The model under review builds one solid part; all positions refer to its coordinate system, in mm. A direction names the side the tool comes from. Round coordinates to 2 decimals unless told otherwise and drop trailing zeros. Order: outer loops, then holes, each group sorted by start corner. A loop starts at its lowest first (then second) coordinate and runs counter-clockwise, first axis right, second up.
```python
from build123d import *

# Parameters (mm, degrees)
SKETCH1_W                  = 44.45
SKETCH1_H                  = 60
CUT_EXTRUDE1_DEPTH         = 50
F_4_CLEARANCE_HOLE1_D      = 3.3
F_4_CLEARANCE_HOLE1_DEPTH  = 8
F_2_CLEARANCE_HOLE1_REACH  = 117.544
F_2_CLEARANCE_HOLE1_BORE_R = 1.25
F_2_CLEARANCE_HOLE2_REACH  = 117.544
F_2_CLEARANCE_HOLE2_BORE_R = 1.25


with BuildPart() as part:
    # Sketch1 → Revolve1 (revolve)
    with BuildSketch(Plane.XZ, mode=Mode.PRIVATE) as revolve1_sk:
        with Locations((22.225, 30)):
            Rectangle(SKETCH1_W, SKETCH1_H)
    revolve(revolve1_sk.sketch.rotate(Axis((0, 0, 60), (0, 0, -1)), 180), axis=Axis((0, 0, 60), (0, 0, -1)))

    # Sketch2 → Cut-Extrude1 (cut)
    with BuildSketch(Plane(origin=(0, 0, 0), x_dir=(-1, 0, 0), z_dir=(0, 0, -1))):
        with BuildLine():
            Line((43.7241638, 8), (43.7241638, -8))
            ThreePointArc((43.7241638, -8), (44.45, 0), (43.7241638, 8))
        make_face()
    extrude(amount=-CUT_EXTRUDE1_DEPTH, mode=Mode.SUBTRACT)

    # Sketch3 → Cut-Revolve1 (revolve, cut)
    with BuildSketch(Plane.XZ, mode=Mode.PRIVATE) as cut_revolve1_sk:
        Polygon((37.5, 60), (0, 60), (0, 0), (37.5, 0), (37.5, 20.5), (32, 20.5), (32, 39.5), (37.5, 39.5), align=None)
    revolve(cut_revolve1_sk.sketch.rotate(Axis((0, 0, 60), (0, 0, -1)), 180), axis=Axis((0, 0, 60), (0, 0, -1)), mode=Mode.SUBTRACT)

    # #4 Clearance Hole1
    with Locations(Plane.XY.offset(60)):
        with Locations((28.991378029, 28.991378029), (0, 41), (-28.991378029, 28.991378029), (-41, 0), (-28.991378029, -28.991378029), (0, -41), (28.991378029, -28.991378029), (41, 0)):
            Hole(F_4_CLEARANCE_HOLE1_D / 2, depth=F_4_CLEARANCE_HOLE1_DEPTH)

    # #2 Clearance Hole1 bore → #2 Clearance Hole1 (cut, up to next)
    with BuildSketch(Plane.ZY.offset(43.7241638), mode=Mode.PRIVATE) as f_2_clearance_hole1_sk1:
        with Locations((15.584748033, 5.15)):
            Circle(F_2_CLEARANCE_HOLE1_BORE_R)
    f_2_clearance_hole1_tool1 = extrude(f_2_clearance_hole1_sk1.sketch, amount=-F_2_CLEARANCE_HOLE1_REACH, mode=Mode.PRIVATE) & part.part
    add(f_2_clearance_hole1_tool1.solids().sort_by_distance((-43.724164, 5.15, 15.584748))[0], mode=Mode.SUBTRACT)

    # #2 Clearance Hole2 bore → #2 Clearance Hole2 (cut, up to next)
    with BuildSketch(Plane.ZY.offset(43.7241638), mode=Mode.PRIVATE) as f_2_clearance_hole2_sk1:
        with Locations((37.834748033, -5.05)):
            Circle(F_2_CLEARANCE_HOLE2_BORE_R)
    f_2_clearance_hole2_tool1 = extrude(f_2_clearance_hole2_sk1.sketch, amount=-F_2_CLEARANCE_HOLE2_REACH, mode=Mode.PRIVATE) & part.part
    add(f_2_clearance_hole2_tool1.solids().sort_by_distance((-43.724164, -5.05, 37.834748))[0], mode=Mode.SUBTRACT)


solid = part.part
```
(1) Consider section C-C (z = 35). Write out the cut boundary in (x, y), and give its area (3 significant figures).
Data:
outline: (-43.72, -8) arc R44.45 ccw (long way) to (-43.72, 8) - close; hole circle Ø64 at (0, 0)
area: 2,980 mm2
(2) Consider section A-A (y = 0). Write out the cut boundary in (x, z).
Data:
outline: (-44.45, 50) - (-43.72, 50) - (-43.72, 0) - (-37.5, 0) - (-37.5, 20.5) - (-32, 20.5) - (-32, 39.5) - (-37.5, 39.5) - (-37.5, 60) - (-39.35, 60) - (-39.35, 52) - (-42.65, 52) - (-42.65, 60) - (-44.45, 60) - close; (32, 20.5) - (37.5, 20.5) - (37.5, 0) - (44.45, 0) - (44.45, 60) - (42.65, 60) - (42.65, 52) - (39.35, 52) - (39.35, 60) - (37.5, 60) - (37.5, 39.5) - (32, 39.5) - close
(3) Consider section B-B (x = -17). Write out the cut boundary in (y, z).
Data:
outline: (-41.07, 0) - (-33.43, 0) - (-33.43, 20.5) - (-27.11, 20.5) - (-27.11, 39.5) - (-33.43, 39.5) - (-33.43, 60) - (-41.07, 60) - close; (27.11, 20.5) - (33.43, 20.5) - (33.43, 0) - (41.07, 0) - (41.07, 60) - (33.43, 60) - (33.43, 39.5) - (27.11, 39.5) - close
(4) Draft analysis for pull direction X (two halves, no side actions). For faces 1 (the cylindrical face through (-37.635, -4.995, 36.586)), 2 (the cylindrical face through (29.35, 27.38, 55.94)), 3 (the flat face through (-43.724, 0, 25)), state which applies: pulls with the +X half, pulls with the -X half, needs draft (parallel to the pull), parting line crosses it, or undercut.
Data:
face 1: needs draft
face 2: undercut
face 3: pulls with the -X half
(5) Insertion check: pin 1 (4.5 mm diameter, centred on x = 41, y = 0, fed in from +Z); pin 2 (1 mm diameter, centred on x = 17.5, z = 18.5, fed in from -Y); pin 3 (1.6 mm diameter, centred on x = -29, y = -29, fed in from +Z); pin 4 (1 mm diameter, centred on x = -3.5, y = 31, fed in from +Z). Each pin has a flat end and moves straight along its axis. Give the tip position at first contact, or say it passes through.
Data:
pin 1: stops at z = 60
pin 2: stops at y = -41.07
pin 3: stops at z = 52
pin 4: passes through
(6) For faces 4 (the flat face through (-32, -20, 0)), 5 (the cylindrical face through (-17.3, -33.27, 10.39)), 6 (the cylindrical face through (-0.89, -39.61, 55.94)), list the 3-axis set-ups (+Z, -Z, +X, -X, +Y, -Y) from which the entire face can be reached by the end or side of a thin tool; tool diameter is ignored.
Data:
face 4: -Z, +X, -X, +Y, -Y
face 5: -Z
face 6: +Z
(7) Consider section D-D (y = 41). Write out the cut boundary in (x, z), and give its area (3 significant figures).
Data:
outline: (-17.17, 0) - (17.17, 0) - (17.17, 60) - (1.65, 60) - (1.65, 52) - (-1.65, 52) - (-1.65, 60) - (-17.17, 60) - close
area: 2,030 mm2
(8) To check wall thickness, follow probe 1 along Z at (x, y) = (-36.75, -5.05); probe 2 along Z at (x, y) = (11, 31.5); probe 3 along Y at (x, z) = (0, 15.25). State the ranges of each line that lie inside material, in increasing order.
Data:
probe 1: z = 20.5 to 36.58, 39.08 to 39.5
probe 2: z = 20.5 to 39.5
probe 3: y = -44.45 to -37.5, 37.5 to 44.45
